Part model, mm, in its own coordinate system. A direction names the side the tool comes from. Coordinates: 2 decimals unless noted, no trailing zeros. Loops run counter-clockwise (first coordinate to the right, second up) from the corner with the lowest first, then second, coordinate; pieces in that order, holes last. Notation, with made-up numbers: (6, -19) - (32, -19) arc R12 ccw to (32, -4) - close; hole circle Ø3 at (57, 33.25). An arc over 180 degrees is marked (long way). Use a Markdown table: item, result. Add a question column.
1) Band-saw the part on C-C (z = -38.25). Give the cut face in (x, y).
2) Band-saw the part on B-B (y = 2.5). Give the cut face in (x, z).
3) Band-saw the part on A-A (y = -7). Give the cut face in (x, z), plus the area to 3 significant figures.
4) Pull direction X, two halves, no side cores. Call faces 6 (the face through (-47, 10, -1)), 7 (the face through (-33.066, 7.535, 75.585)), 8 (the face through (-23.735, -7.918, 0.522)), 9 (the face through (-92.778, 7.465, 2.041)): +X half, -X half, draft (parallel to the pull), parting line (faces both ways), or undercut.
5) Drop flat-ended pins along their axis: P1, Ø8, axis at x = -11.5, y = 0.5, coming from the +Z side; P2, Ø12, axis at y = -10.5, z = -35, coming from the -X side; P3, Ø5.5, axis at x = -1.5, y = 1.5, coming from the +Z side. Give the stop position or say it passes through.
6) Band-saw the part on D-D (x = -55.5). Give the cut face in (y, z).
7) Tool access for faces 1 (the face through (-2, 2, -47.25)), 2 (the face through (-28.735, -7.918, 0.567)), 3 (the face through (-3, 2, 47.25)), 4 (the face through (-26, -20, -4)), 5 (the face through (0, -2, -41)): list every direction of +Z, -Z, +X, -X, +Y, -Y with a clear straight run to the whole face (end or side of a thin tool).
8) Probe probe 1 along Y at (x, z) = (-44, -6); probe 2 along X at (y, z) = (-7.5, -44); probe 3 along Z at (x, y) = (-14, -9.5). List the from-to ranges inside material, lowest first. Write a range as [from, to].
Autodesk Inventor part; units mm, degrees
ref_plane "YZ Plane" through (0, 0, 0) normal (1, 0, 0) x (0, 1, 0)
ref_plane "XZ Plane" through (0, 0, 0) normal (0, 1, 0) x (-1, 0, 0)
ref_plane "XY Plane" through (0, 0, 0) normal (0, 0, 1) x (1, 0, 0)
sketch "Skizze1" plane through (0, 0, 0) normal (0, 1, 0) x (-1, 0, 0)
  circle A0 centre (0, 0) radius 22.25
  circle A1 centre (0, 0) radius 27.25
  line L0 (5, 47.25) -> (-5, 47.25)
  line L1 (-5, 47.25) -> (-5, -47.25)
  line L2 (-5, -47.25) -> (5, -47.25)
  line L3 (5, -47.25) -> (5, 47.25)
  line L4 (5, 47.25) -> (-5, -47.25) construction
  line L5 (-5, 47.25) -> (5, -47.25) construction
  line L6 (0, 47.25) -> (0, -47.25)
  point P0 (0, 22.25)
  point P1 (0, -22.25)
  point P2 (5, -26.7874)
  point P3 (5, 26.7874)
  dimension "d0" = 44.5
  dimension "d1" = 54.5
  dimension "d2" = 10
  dimension "d3" = 94.5
extrude "Extrusion1" add sketch "Skizze1" along normal blind 5 contours A0 L3 A1 | A0 L6 A1 L3 | L3 A1 L6 A0 | A1 L6 L0 L3 | L3 L2 L6 A1
sketch "Skizze4" plane through (0, 5, 0) normal (0, 1, 0) x (1, 0, 0)
  circle A0 centre (0, 0) radius 22.25
  circle A1 centre (0, 0) radius 92.8
  circle A2 centre (0, 0) radius 72.8
  line L0 (0, -92.8) -> (0, 92.8)
  point P0 (0, 22.25)
  point P1 (0, -22.25)
  dimension "d23" = 185.6
  dimension "d24" = 145.6
  dimension "d43" = 44.5
extrude "Extrusion4" add sketch "Skizze4" along normal blind 5 contours A0 L0 A2 | A2 L0 A1 picked at (-55.7302, 0.894) picked at (-74.476, -42.8466)
sketch "Skizze5" plane through (0, 10, 0) normal (0, 1, 0) x (1, 0, 0)
  circle A0 centre (0, 0) radius 52.8
  arc A1 (0, 92.8) -> (0, -92.8) centre (0, 0) ccw
  line L0 (0, 0) -> (72.8, 0) construction
  line L1 (0, 0) -> (72.8, 0) construction
  circle A2 centre (0, 0) radius 85.3
  line L2 (0, 0) -> (-35.513, 85.736)
  line L3 (0, 0) -> (92.8, 0) construction
  line L4 (0, 0) -> (-85.736, 35.513)
  line L5 (0, 0) -> (92.8, 0) construction
  line L6 (0, 0) -> (-35.513, -85.736)
  line L7 (0, 0) -> (92.8, 0) construction
  line L8 (0, 0) -> (-85.736, -35.513)
  line L9 (0, 0) -> (92.8, 0) construction
  circle A3 centre (-32.6429, -78.8069) radius 3.25
  circle A4 centre (-78.8069, -32.6429) radius 3.25
  circle A5 centre (-78.8069, 32.6429) radius 3.25
  circle A6 centre (-32.6429, 78.8069) radius 3.25
  circle A7 centre (0, 0) radius 77.8
  dimension "d27" = 105.6
  dimension "d31" = 170.6
  dimension "d32" = 112.5
  dimension "d33" = 157.5
  dimension "d34" = 112.5
  dimension "d35" = 157.5
  dimension "d36" = 6.5
  dimension "d37" = 6.5
  dimension "d38" = 6.5
  dimension "d39" = 6.5
  dimension "d42" = 155.6
extrude "Extrusion5" cut sketch "Skizze5" against normal through all contours A6 A2 L2 | L2 A2 A6 | A3 A2 L6 | L6 A2 A3 | A5 A2 L4 | L4 A2 A5 | L2 A6 A2 | A2 A6 L2 | A4 A2 L8 | L8 A2 A4 | L6 A3 A2 | A2 A3 L6 | L4 A5 A2 | A2 A5 L4 | L8 A4 A2 | A2 A4 L8
sketch "Skizze6" plane through (0, 0, 0) normal (0, -1, 0) x (1, 0, 0)
  circle A0 centre (0, 0) radius 38.25
  line L0 (5, 63.25) -> (-5, 63.25)
  line L1 (-5, 63.25) -> (-5, -63.25)
  line L2 (-5, -63.25) -> (5, -63.25)
  line L3 (5, -63.25) -> (5, 63.25)
  line L4 (5, 63.25) -> (-5, -63.25) construction
  line L5 (-5, 63.25) -> (5, -63.25) construction
  circle A1 centre (0, 0) radius 43.25
  circle A2 centre (0, 0) radius 22.25
  line L6 (0, -47.25) -> (0, -92.8)
  line L7 (0, -63.25) -> (0, 63.25)
  point P0 (-5, 42.96)
  point P1 (-5, -42.96)
  point P2 (0, -22.25)
  point P3 (0, 22.25)
  dimension "d44" = 76.5
  dimension "d45" = 10
  dimension "d46" = 126.5
  dimension "d47" = 86.5
extrude "Extrusion6" add sketch "Skizze6" along normal blind 85 contours L7 A2 L1 A0 | A0 L1 A1 L7 | L7 A1 L1 A0 | A0 L1 A2 L7 | L1 A2 A0 | A0 L1 A1 | A1 L1 L0 L7 | L7 L6 L2 L1 A1
chamfer "Fasen1" distance 16 distance2 85 1 edges at (-22.25, -85, 0) measured on face at (-1.6667, -85, -42.82)
chamfer "Fasen2" distance 85 angle 10.66 1 edges at (-2.5, 0, -63.25) measured on face at (-3.3333, -28.3333, -63.25)
chamfer "Fasen3" distance 85 distance2 16 1 edges at (-2.5, 0, 63.25) measured on face at (-1.6667, -28.3333, 63.25)
chamfer "Fasen4" distance 85 distance2 16 1 edges at (-43.25, 0, 0) measured on face at (-38.2627, -56.6667, -20.1626)
sketch "Skizze7" plane through (0, -85, 0) normal (0, -1, 0) x (1, 0, 0)
  circle A0 centre (0, 0) radius 65
  dimension "d62" = 130
extrude "Extrusion7" cut sketch "Skizze7" against normal blind 65
sketch "Skizze8" plane through (-5, 5, -47.25) normal (-1, 0, 0) x (0, 0, 1)
  circle A0 centre (9, -12) radius 3.25
  line L0 (-3.7651, -25) -> (16.641, -25)
  line L1 (0, -5) -> (0, 0)
  point P0 (47.25, -5)
  dimension "d65" = 6.5
  dimension "d66" = 13
  dimension "d67" = 9
sketch "Skizze9" plane through (-5, 5, 26.7874) normal (-1, 0, 0) x (0, 0, 1)
  circle A0 centre (11.4626, -12) radius 3.25
  line L0 (3.8217, -25) -> (24.2273, -25)
  line L1 (20.4626, -5) -> (20.4626, 0)
  point P0 (-26.7874, -5)
  dimension "d68" = 6.5
  dimension "d69" = 13
  dimension "d70" = 9
extrude "Extrusion8" cut sketch "Skizze8" against normal through all
extrude "Extrusion9" cut sketch "Skizze9" against normal through all
properties part number "rohr-mount-v2"
Answer block:
| question | item | result |
|---|---|---|
| 1 | outline | (-84.55, 5) - (-5, 5) - (-5, -3.75) - (0, -3.75) - (0, 10) - (-84.55, 10) - close; (-5, -20) - (0, -20) - (0, -10.25) - (-5, -10.25) - close |
| 2 | outline | (-5, -47.25) - (0, -47.25) - (0, -22.25) arc R22.25 cw to (0, 22.25) - (0, 47.25) - (-5, 47.25) - (-5, 26.79) arc R27.25 ccw to (-5, -26.79) - close |
| 3 | outline | (-5, -48.57) - (0, -48.57) - (0, -41.5) - (-5, -41.5) - close; (-5, -35) - (0, -35) - (0, -23.57) arc R23.57 cw to (0, 23.57) - (0, 35) - (-5, 35) - (-5, 28.13) arc R28.57 ccw to (-5, -28.13) - close; (-5, 41.5) - (0, 41.5) - (0, 48.57) - (-5, 48.57) - close |
| 3 | area | 546 mm2 |
| 4 | face 6 | draft |
| 4 | face 7 | undercut |
| 4 | face 8 | +X half |
| 4 | face 9 | -X half |
| 5 | P1 | z = 26.34 |
| 5 | P2 | x = -5 |
| 5 | P3 | z = 47.49 |
| 6 | outline | (5, -74.37) - (10, -74.37) - (10, 74.37) - (5, 74.37) - close |
| 7 | face 1 | -Z, +X, -X |
| 7 | face 2 | -X |
| 7 | face 3 | +Z, +X, -X |
| 7 | face 4 | +Z, -Z, +X, -X, -Y |
| 7 | face 5 | +Z, -Z, +X, +Y, -Y |
| 8 | probe 1 | [5, 10] |
| 8 | probe 2 | [-5, 0] |
| 8 | probe 3 | [-25.44, -19.54], [19.54, 25.44] |
